The listing builds one solid part. Answer for the finished solid, in the listing's coordinates (mm). A direction names the side the tool comes from. Coordinates: 2 decimals unless noted, no trailing zeros. Loops run counter-clockwise (first coordinate to the right, second up) from the corner with the lowest first, then second, coordinate; pieces in that order, holes last. Notation, with made-up numbers: (69.25, 86) - (96.25, 86) arc R17 ccw to (96.25, 104) - close; hole circle Ø7 at (-21, -10). An arc over 180 degrees is marked (long way). Write each question's results on one line, items separated by ' | '. Start each with the question number.
(1) Find section A-A on z = -6.5. Determine the outline of the cut face in (x, y).
(2) Find section B-B on y = 1. Determine the outline of the cut face in (x, z) (3 decimals).
(3) For faces 1 (the flat face through (17.526, 31, 0)), 2 (the flat face through (0, -12.7, -6)), 3 (the flat face through (-1, 31.75, 0)), determine the directions among +Z, -Z, +X, -X, +Y, -Y from which every point of the face is accessible in a straight line to the end or side of a thin tool.
(4) Determine the mould class of faces 4 (the flat face through (19, -31, 1.524)), 5 (the flat face through (-31, 19.05, 1)), 6 (the flat face through (0, 0, -0.635)) for opening direction Z: released by +Z, released by -Z, zero draft, split by the parting line, or undercut.
(5) Find section C-C on x = -1. Determine the outline of the cut face in (y, z) (3 decimals).
(6) Given pin 1 Ø8 at (x, y) = (16, -13.5) entering from +Z (3 decimals); pin 2 Ø4 at (x, y) = (30.5, 26) entering from +Z (3 decimals), each flat-ended and moving along its own axis, determine where each tip first touches the part or whether it passes through.
(7) Find section D-D on z = 6. Determine the outline of the cut face in (x, y), then the cut area to 3 significant figures.
(8) Consider line 1 (X direction, y = 25, z = -1.5); line 2 (X direction, y = 2, z = -9); line 3 (Y direction, x = 14.5, z = 3). Determine where each line is inside the solid, lowest interval first. Write a range as from..to.
from build123d import *

# Parameters (mm, degrees)
F0_W      = 76.2
F0_H      = 34.29
F1_DEPTH  = 31.75
F2_W      = 72.039268
F2_H      = 59.124664
F3_DEPTH  = 33.02
F4_W      = 3.048
F4_H      = 1.524
F5_DEPTH  = 76.2
F7_DEPTH  = 33.02
F8_W      = 25.4
F8_H      = 25.4
F9_DEPTH  = 20.32
F10_W     = 25.4
F10_H     = 15.1343
F11_DEPTH = 5.08


with BuildPart() as f1:
    # F0 (on Front) → F1 (new body, symmetric)
    with BuildSketch(Plane.XZ):
        Rectangle(F0_W, F0_H)
    extrude(amount=F1_DEPTH, both=True)

    # F2 (on face) → F3 (cut)
    with BuildSketch(Plane.XY.offset(17.145)):
        Rectangle(F2_W, F2_H)
    extrude(amount=-F3_DEPTH, mode=Mode.SUBTRACT)

    # F4 (on face) → F5 (cut)
    with BuildSketch(Plane.XZ.offset(31.75)):
        with Locations((-19.05, 0.762)):
            Rectangle(F4_W, F4_H)
        with Locations((19.05, 0.762)):
            Rectangle(F4_W, F4_H)
        with Locations((19.05, -0.762)):
            Rectangle(F4_W, F4_H)
        with Locations((-19.05, -0.762)):
            Rectangle(F4_W, F4_H)
    extrude(amount=-F5_DEPTH, mode=Mode.SUBTRACT)

    # F6 (on face) → F7 (join)
    with BuildSketch(Plane.XY.offset(17.145)):
        with BuildLine():
            Line((-34.578427, 28.228427), (-38.1, 31.75))
            Line((-38.1, 31.75), (-38.1, 19.05))
            Line((-38.1, 19.05), (-25.4, 19.05))
            Line((-25.4, 19.05), (-28.921573, 22.571573))
            ThreePointArc((-28.921573, 22.571573), (-34.578427, 22.571573), (-34.578427, 28.228427))
        make_face()
        with BuildLine():
            Line((-25.4, 31.75), (-38.1, 31.75))
            Line((-38.1, 31.75), (-34.578427, 28.228427))
            ThreePointArc((-34.578427, 28.228427), (-30.219266, 29.095518), (-27.75, 25.4))
            ThreePointArc((-27.75, 25.4), (-28.054482, 23.869266), (-28.921573, 22.571573))
            Line((-28.921573, 22.571573), (-25.4, 19.05))
            Line((-25.4, 19.05), (-25.4, 31.75))
        make_face()
        with BuildLine():
            Line((-34.578427, -28.228427), (-38.1, -31.75))
            Line((-38.1, -31.75), (-25.4, -31.75))
            Line((-25.4, -31.75), (-25.4, -19.05))
            Line((-25.4, -19.05), (-28.921573, -22.571573))
            ThreePointArc((-28.921573, -22.571573), (-28.054482, -23.869266), (-27.75, -25.4))
            ThreePointArc((-27.75, -25.4), (-30.219266, -29.095518), (-34.578427, -28.228427))
        make_face()
        with BuildLine():
            Line((-38.1, -19.05), (-38.1, -31.75))
            Line((-38.1, -31.75), (-34.578427, -28.228427))
            ThreePointArc((-34.578427, -28.228427), (-34.578427, -22.571573), (-28.921573, -22.571573))
            Line((-28.921573, -22.571573), (-25.4, -19.05))
            Line((-25.4, -19.05), (-38.1, -19.05))
        make_face()
        with BuildLine():
            Line((34.578427, -28.228427), (38.1, -31.75))
            Line((38.1, -31.75), (38.1, -19.05))
            Line((38.1, -19.05), (25.4, -19.05))
            Line((25.4, -19.05), (28.921573, -22.571573))
            ThreePointArc((28.921573, -22.571573), (33.280734, -21.704482), (35.75, -25.4))
            ThreePointArc((35.75, -25.4), (35.445518, -26.930734), (34.578427, -28.228427))
        make_face()
        with BuildLine():
            Line((25.4, -31.75), (38.1, -31.75))
            Line((38.1, -31.75), (34.578427, -28.228427))
            ThreePointArc((34.578427, -28.228427), (28.921573, -28.228427), (28.921573, -22.571573))
            Line((28.921573, -22.571573), (25.4, -19.05))
            Line((25.4, -19.05), (25.4, -31.75))
        make_face()
        with BuildLine():
            Line((34.578427, 28.228427), (38.1, 31.75))
            Line((38.1, 31.75), (25.4, 31.75))
            Line((25.4, 31.75), (25.4, 19.05))
            Line((25.4, 19.05), (28.921573, 22.571573))
            ThreePointArc((28.921573, 22.571573), (28.921573, 28.228427), (34.578427, 28.228427))
        make_face()
        with BuildLine():
            Line((38.1, 19.05), (38.1, 31.75))
            Line((38.1, 31.75), (34.578427, 28.228427))
            ThreePointArc((34.578427, 28.228427), (35.445518, 26.930734), (35.75, 25.4))
            ThreePointArc((35.75, 25.4), (33.280734, 21.704482), (28.921573, 22.571573))
            Line((28.921573, 22.571573), (25.4, 19.05))
            Line((25.4, 19.05), (38.1, 19.05))
        make_face()
    extrude(amount=-F7_DEPTH)

    # F8 (on face) → F9 (join)
    with BuildSketch(Plane.XY.offset(-15.875)):
        Rectangle(F8_W, F8_H)
    extrude(amount=F9_DEPTH)

    # F10 (on face) → F11 (cut)
    with BuildSketch(Plane.XY.offset(4.445)):
        Rectangle(F10_W, F10_H)
    extrude(amount=-F11_DEPTH, mode=Mode.SUBTRACT)


solid = f1.part
Values:
1) outline: (-38.1, -31.75) - (38.1, -31.75) - (38.1, 31.75) - (-38.1, 31.75) - close; (-12.7, -12.7) - (12.7, -12.7) - (12.7, 12.7) - (-12.7, 12.7) - close; hole (-36.02, -19.05) - (-25.4, -19.05) - (-25.4, -29.56) - (25.4, -29.56) - (25.4, -19.05) - (36.02, -19.05) - (36.02, 19.05) - (25.4, 19.05) - (25.4, 29.56) - (-25.4, 29.56) - (-25.4, 19.05) - (-36.02, 19.05) - close; hole circle Ø8 at (-31.75, -25.4); hole circle Ø8 at (-31.75, 25.4); hole circle Ø8 at (31.75, -25.4); hole circle Ø8 at (31.75, 25.4)
2) outline: (-38.1, -17.145) - (38.1, -17.145) - (38.1, 17.145) - (36.02, 17.145) - (36.02, -15.875) - (12.7, -15.875) - (12.7, -0.635) - (-12.7, -0.635) - (-12.7, -15.875) - (-36.02, -15.875) - (-36.02, 17.145) - (-38.1, 17.145) - close
3) face 1: +Y, -Y | face 2: +Z | face 3: +Z, -Z, +X, -X, +Y
4) face 4: undercut | face 5: zero draft | face 6: released by +Z
5) outline: (-31.75, -17.145) - (31.75, -17.145) - (31.75, 17.145) - (29.562, 17.145) - (29.562, -15.875) - (12.7, -15.875) - (12.7, 4.445) - (7.567, 4.445) - (7.567, -0.635) - (-7.567, -0.635) - (-7.567, 4.445) - (-12.7, 4.445) - (-12.7, -15.875) - (-29.562, -15.875) - (-29.562, 17.145) - (-31.75, 17.145) - close
6) pin 1: stops at z = 4.445 | pin 2: stops at z = -15.875
7) outline: (-38.1, -31.75) - (38.1, -31.75) - (38.1, 31.75) - (-38.1, 31.75) - close; hole (-36.02, -19.05) - (-25.4, -19.05) - (-25.4, -29.56) - (25.4, -29.56) - (25.4, -19.05) - (36.02, -19.05) - (36.02, 19.05) - (25.4, 19.05) - (25.4, 29.56) - (-25.4, 29.56) - (-25.4, 19.05) - (-36.02, 19.05) - close; hole circle Ø8 at (-31.75, -25.4); hole circle Ø8 at (-31.75, 25.4); hole circle Ø8 at (31.75, -25.4); hole circle Ø8 at (31.75, 25.4) | area: 825 mm²
8) line 1: x = -38.1..-35.73, -27.77..-25.4, 25.4..27.77, 35.73..38.1 | line 2: x = -38.1..-36.02, -12.7..12.7, 36.02..38.1 | line 3: y = -31.75..-29.56, 29.56..31.75
